from build123d import *

# Parameters (mm, degrees)
BOSS_EXTRUDE1_DEPTH = 6.4


with BuildPart() as part:
    # Sketch1 → Boss-Extrude1 (new body)
    with BuildSketch(Plane(origin=(0, 0, 0), x_dir=(0, 0, -1), z_dir=(1, 0, 0))):
        Polygon((7.699451661, 16.299320413), (7.699451661, 15.050679587), (-0.190789953, 15.050679587), (-0.190789953, 26.875784077), (-5.692060153, 27.152292188), (-5.689519376, 36.852291855), (-0.190789953, 37.125784431), (-0.190789953, 45.489990555), (55.075, 45.489990555), (55.075, 55.887449255), (57.075, 57.887449255), (70.079421798, 57.887449255), (70.115, 52.889990555), (63.115, 50.9), (63.115, 45.489442951), (153.305, 45.490143945), (153.305, 55.887449255), (155.305, 57.887449255), (168.309421798, 57.887449255), (168.345, 52.889990555), (161.345, 50.9), (161.345, 45.489442951), (186.745000058, 45.489442951), (186.748098344, 0), (136.598098344, 0), (136.598098344, 7.7113021), (137.848098344, 7.7113021), (137.848098344, 9.5113021), (136.598098344, 9.5113021), (136.598098344, 10.9113021), (133.59673917, 10.9113021), (133.59673917, 9.5113021), (132.348098344, 9.5113021), (132.348098344, 7.7113021), (133.59673917, 7.7113021), (133.59673917, 0), (118.842364298, 0), (73.842364298, 0), (0, 0), (-0.190789953, 0.087763288), (-0.190789953, 12.049320413), (7.699451661, 12.049320413), (7.699451661, 10.799320413), (9.499451661, 10.799320413), (9.499451661, 12.049320413), (10.899451661, 12.049320413), (10.899451661, 15.050679587), (9.499451661, 15.050679587), (9.499451661, 16.299320413), align=None)
        Polygon((60.842364298, 5), (127.342364298, 5), (127.342364298, 24), (121.342364298, 30), (66.842364298, 30), (60.842364298, 24), align=None, mode=Mode.SUBTRACT)
    extrude(amount=BOSS_EXTRUDE1_DEPTH)


solid = part.part
Geometry: final body of the model. Coordinates: model frame, mm. A direction names the side the tool comes from. Round coordinates to 2 decimals unless told otherwise and drop trailing zeros. Write each loop counter-clockwise with the first axis right and the second up, starting at its lowest first coordinate (ties: lowest second). Pieces come first, ordered by that corner, then holes. Notation, with made-up numbers: M 88,3 L 129,3 A28 cw 129,22 Z; hole C 3.25,-34.75 d11. An arc over 180 degrees is marked long. Write item = value, one per line.
Item 1: Section query C-C on z = -40. Return loops of the section in (x, y), then the cut area to 3 significant figures.
Findings:
outline = M 0,0 L 6.4,0 L 6.4,45.49 L 0,45.49 Z
area = 291 mm^2
Item 2: Access query for faces 4 (the face through (3, 48, -63.115)), 5 (the face through (3, 45.49, -27)), 6 (the face through (3, 4, -133.597)), 7 (the face through (3, 21, 0.191)), 8 (the face through (3, 15.051, -4)). Directions: +Z, -Z, +X, -X, +Y, -Y. A direction counts if a zero-diameter tool reaches every point of the face in a straight line with its end or side. Return the directions, or none.
Findings:
face_4 = +X, -X
face_5 = +Z, +X, -X, +Y
face_6 = +X, -X, -Y
face_7 = +Z, +X, -X, -Y
face_8 = +Z, +X, -X
Item 3: Material intervals for line 1 along Z through (x, y) = (4.25, 11.5); line 2 along Z through (x, y) = (2.5, 15); line 3 along Z through (x, y) = (2.75, 47.5) (3 decimals), sorted ascending. Write a range as [from, to].
Findings:
line_1 = [-186.75, -127.34], [-60.84, -9.5], [-7.7, 0.19]
line_2 = [-186.75, -127.34], [-60.84, -10.9]
line_3 = [-161.345, -153.305], [-63.115, -55.075]
Item 4: Section query A-A on z = -82.5. Return loops of the section in (x, y), then the cut area to 3 significant figures.
Findings:
outline = M 0,0 L 6.4,0 L 6.4,5 L 0,5 Z; M 0,30 L 6.4,30 L 6.4,45.49 L 0,45.49 Z
area = 131 mm^2
Item 5: Pull-direction query (Z, two-part tool) for faces 1 (the face through (3, 51, -153.305)), 2 (the face through (3, 12.049, -4)), 3 (the face through (3, 48, -161.345)); classes: pulls with the +Z half, pulls with the -Z half, needs draft (parallel to the pull), parting line crosses it, or undercut.
Findings:
face_1 = undercut
face_2 = needs draft
face_3 = pulls with the -Z half
Item 6: Pin query (flat end, axial travel): P1, Ø1.5, axis at x = 2.5, z = -134.5, coming from the -Y side; P2, Ø1.5, axis at y = 47, z = -109.5, coming from the +X side; P3, Ø5, axis at y = 7.5, z = -147, coming from the -X side; P4, Ø3, axis at x = 4.5, y = 41.5, coming from the +Z side. Return the tip coordinate at first contact, or that it passes through.
Findings:
P1 = 10.91
P2 = through
P3 = 0
P4 = 0.19
Item 7: Section query B-B on y = 21. Return loops of the section in (x, z).
Findings:
outline = M 0,-186.75 L 6.4,-186.75 L 6.4,-127.34 L 0,-127.34 Z; M 0,-60.84 L 6.4,-60.84 L 6.4,0.19 L 0,0.19 Z
